Autodesk Inventor part; units mm, degrees
ref_plane "YZ Plane" through (0, 0, 0) normal (1, 0, 0) x (0, 1, 0)
ref_plane "XZ Plane" through (0, 0, 0) normal (0, 1, 0) x (-1, 0, 0)
ref_plane "XY Plane" through (0, 0, 0) normal (0, 0, 1) x (1, 0, 0)
sketch "スケッチ1" plane through (0, 0, 0) normal (0, 0, 1) x (1, 0, 0)
  circle A0 centre (0, 0) radius 2.5
  circle A1 centre (0, 0) radius 6
  circle A2 centre (0, 0) radius 9.5
  circle A3 centre (0, 7.5) radius 1
  circle A4 centre (0, 0) radius 7.5 construction
  line L0 (0, -20.3) -> (0, 20.3)
  circle A5 centre (-6.4952, -3.75) radius 1
  circle A6 centre (6.4952, -3.75) radius 1
  circle A7 centre (0, 0) radius 14.5 construction
  line L1 (-7, 6.4226) -> (-7, 10.9226)
  line L2 (-6, 11.9226) -> (6, 11.9226)
  line L3 (7, 10.9226) -> (7, 6.4226)
  arc A8 (-6, 11.9226) -> (-7, 10.9226) centre (-6, 10.9226) ccw
  arc A9 (7, 10.9226) -> (6, 11.9226) centre (6, 10.9226) ccw
  circle A10 centre (5.25, 10.2317) radius 2 construction
  circle A11 centre (5.25, 10.2317) radius 0.8
  circle A12 centre (-5.25, 10.2317) radius 2 construction
  circle A13 centre (-5.25, 10.2317) radius 0.8
  line L4 (-5.25, 10.2317) -> (-5.25, 7.9175) construction
  line L5 (5.25, 10.2317) -> (5.25, 7.9175) construction
  circle A14 centre (5.25, -10.2317) radius 0.8
  line L6 (7, -6.4226) -> (7, -10.9226)
  arc A15 (6, -11.9226) -> (7, -10.9226) centre (6, -10.9226) ccw
  line L7 (6, -11.9226) -> (-6, -11.9226)
  circle A16 centre (-5.25, -10.2317) radius 2 construction
  line L8 (-7, -10.9226) -> (-7, -6.4226)
  arc A17 (-7, -10.9226) -> (-6, -11.9226) centre (-6, -10.9226) ccw
  circle A18 centre (-5.25, -10.2317) radius 0.8
  circle A19 centre (5.25, -10.2317) radius 2 construction
  dimension "d4" = 15
  dimension "d0" = 5
  dimension "d1" = 12
  dimension "d2" = 19
  dimension "d3" = 2
  dimension "d7" = 360
  dimension "d13" = 29
  dimension "d14" = 1
  dimension "d15" = 12
  dimension "d16" = 4.5
  dimension "d17" = 4
  dimension "d18" = 1.6
  dimension "d19" = 10.5
  dimension "d22" = 360
extrude "押し出し1" add sketch "スケッチ1" along normal blind 1.25 contours A0 L0 A1 | A0 L0 A1 | L0 A3 A2 A1 | A1 L0 A2 A3
extrude "押し出し2" add sketch "スケッチ1" along normal blind 2.5 contours L0 A3 A2 A1 | A1 L0 A2 A3
extrude "押し出し3" add sketch "スケッチ1" along normal blind 8 contours L0 L7 A17 L8 A2 | A2 L6 A15 L7 L0 | L0 L2 A9 L3 A2 | A2 L1 A8 L2 L0
properties part number "MotorMount_sub"
Input: part model. Units: mm. Frame: model coordinates. A direction names the side the tool comes from. Round coordinates to 2 decimals unless told otherwise and drop trailing zeros. Loops run counter-clockwise (first coordinate to the right, second up) from the corner with the lowest first, then second, coordinate; pieces in that order, holes last. Notation, with made-up numbers: (54.25, 82.25) - (110.25, 82.25) arc R18 cw to (110.25, 90.25) - close; hole circle Ø4 at (-6.75, -37.75). An arc over 180 degrees is marked (long way). One line per item, written item: value. Start each with the question number.
(1) Access query for faces 4 (the flat face through (-7, -9, 4)), 5 (the cylindrical face through (-5.9, 10.7, 3.9)), 6 (the flat face through (7, 9, 4)), 7 (the flat face through (6.2, 0.1, 2.5)). Directions: +Z, -Z, +X, -X, +Y, -Y. A direction counts if a zero-diameter tool reaches every point of the face in a straight line with its end or side. Return the directions, or none.
(2) Section B-B, the plane z = 5.25. Return loops of the section in (x, y), plus the area to 3 significant figures.
(3) Section A-A, the plane y = 0. Return loops of the section in (x, z), plus the area to 4 significant figures.
(4) Ray query, line 1 (Y direction, x = 0, z = 1.9); line 2 (X direction, y = 0, z = 0.6); line 3 (X direction, y = 10, z = 7). Return the intervals inside material, ascending. Write a range as [from, to].
(5) Contact query for flat-ended pins moving along their axis: P1, Ø1.4, axis at x = 5.25, y = -10.23, coming from the -Z side; P2, Ø2, axis at y = 9.5, z = 3.5, coming from the -X side; P3, Ø3.5, axis at x = -2, y = -1, coming from the +Z side; P4, Ø1, axis at x = 2.5, y = 6.5, coming from the +Z side. Output: stop coordinate, or through.
(6) Section C-C, the plane x = -2. Return loops of the section in (y, z).
(7) Section D-D, the plane z = 2. Count the separate pieces of the cut face and the enclosed holes in it, plus the area to 3 significant figures.
(8) Draft query along Y for faces 1 (the cylindrical face through (6.715, -11.622, 3.944)), 2 (the cylindrical face through (4.6, 10.7, 3.9)), 3 (the flat face through (0, -10, 8)). Return one class per face: +Y half, -Y half, draft (parallel to the pull), parting line (faces both ways), or undercut.
Results below:
1. face 4: +Z, -Z, -X, -Y
1. face 5: +Z, -Z
1. face 6: +Z, -Z, +X, +Y
1. face 7: +Z
2. outline: (-7, -10.92) arc R1 ccw to (-6, -11.92) - (6, -11.92) arc R1 ccw to (7, -10.92) - (7, -6.42) arc R9.5 cw to (-7, -6.42) - close; (-7, 6.42) arc R9.5 cw to (7, 6.42) - (7, 10.92) arc R1 ccw to (6, 11.92) - (-6, 11.92) arc R1 ccw to (-7, 10.92) - close; hole circle Ø1.6 at (-5.25, -10.23); hole circle Ø1.6 at (-5.25, 10.23); hole circle Ø1.6 at (5.25, -10.23); hole circle Ø1.6 at (5.25, 10.23)
2. area: 85.5 mm^2
3. outline: (-9.5, 0) - (-2.5, 0) - (-2.5, 1.25) - (-6, 1.25) - (-6, 2.5) - (-9.5, 2.5) - close; (2.5, 0) - (9.5, 0) - (9.5, 2.5) - (6, 2.5) - (6, 1.25) - (2.5, 1.25) - close
3. area: 26.25 mm^2
4. line 1: [-11.92, -6], [6, 6.5], [8.5, 11.92]
4. line 2: [-9.5, -2.5], [2.5, 9.5]
4. line 3: [-7, -6.02], [-4.48, 4.48], [6.02, 7]
5. P1: through
5. P2: x = -7
5. P3: z = 1.25
5. P4: z = 2.5
6. outline: (-11.92, 0) - (-1.5, 0) - (-1.5, 1.25) - (-5.66, 1.25) - (-5.66, 2.5) - (-9.29, 2.5) - (-9.29, 8) - (-11.92, 8) - close; (1.5, 0) - (11.92, 0) - (11.92, 8) - (9.29, 8) - (9.29, 2.5) - (5.66, 2.5) - (5.66, 1.25) - (1.5, 1.25) - close
7. separate pieces: 1
7. enclosed holes: 8
7. area: 246 mm^2
8. face 1: -Y half
8. face 2: undercut
8. face 3: draft
